Source: CAD feature listing. Evaluate the final solid. Frame: model axes, mm. A direction names the side the tool comes from. Give positions to 0.01 mm unless a question says otherwise; leave off trailing zeros. Order: outer loops, then holes, each group sorted by start corner. A loop starts at its lowest first (then second) coordinate and runs counter-clockwise, first axis right, second up. Notation, with made-up numbers: (76.5, 49.5) - (122.5, 49.5) arc R17 cw to (122.5, 82.5) - close; hole circle Ø4 at (28, -4). An arc over 180 degrees is marked (long way). Write each question's results on one line, items separated by ' | '. Start each with the question number.
Item 1: Section B-B on x = 1.1. Output: boundary loops of the cut face in (y, z).
Item 2: Set-up query: faces 5 (the flat face through (1, -52.5, 23)), 6 (the flat face through (1, -33, -20)). Return all of +Z, -Z, +X, -X, +Y, -Y with unobstructed straight access to the full face (end or side cutting, diameter ignored); none if empty.
Item 3: Section A-A on z = 0. Output: boundary loops of the cut face in (x, y).
Item 4: Section D-D on z = -6.5. Output: boundary loops of the cut face in (x, y), and give its area (3 significant figures).
Item 5: Contact query for flat-ended pins moving along their axis: pin 1 Ø3 at (y, z) = (0, 0) entering from -X; pin 2 Ø1.5 at (x, z) = (1.5, 10.5) entering from -Y. Output: stop coordinate, or through.
Item 6: Mould query, pull axis Z, two halves, no side actions, for faces 1 (the flat face through (1, -27, -25)), 2 (the flat face through (1, -26, 25)), 3 (the cylindrical face through (1.48, -2.44, 0.54)), 4 (the cylindrical face through (1.479, 24.994, -0.55)). Classes: released by +Z, released by -Z, zero draft, split by the parting line, or undercut.
Item 7: Section C-C on y = -33.5. Output: boundary loops of the cut face in (x, z).
Item 8: Line query: line 1 along Y through (x, z) = (2.25, 0); line 2 along Z through (x, y) = (2.2, -16); line 3 along Z through (x, y) = (0.65, -33). Output: solid intervals per line, ascending.
```python
from build123d import *

# Parameters (mm, degrees)
SKETCH1_R           = 2.5
BOSS_EXTRUDE1_DEPTH = 3


with BuildPart() as part:
    # Sketch1 → Boss-Extrude1 (new body)
    with BuildSketch(Plane(origin=(0, 0, 0), x_dir=(0, 0, -1), z_dir=(1, 0, 0))):
        with BuildLine():
            ThreePointArc((-20, -15), (-23.717082451, -7.90569415), (-25, 0))
            Line((-25, 0), (-25, -52.5))
            Line((-25, -52.5), (-20, -52.5))
            Line((-20, -52.5), (-20, -15))
        make_face()
        with BuildLine():
            ThreePointArc((25, 0), (0, 25), (-25, 0))
            ThreePointArc((-25, 0), (-23.717082451, -7.90569415), (-20, -15))
            ThreePointArc((-20, -15), (0, -25), (20, -15))
            ThreePointArc((20, -15), (23.717082451, -7.90569415), (25, 0))
        make_face()
        Circle(SKETCH1_R, mode=Mode.SUBTRACT)
        with BuildLine():
            Line((25, -52.5), (25, 0))
            ThreePointArc((25, 0), (23.717082451, -7.90569415), (20, -15))
            Line((20, -15), (20, -52.5))
            Line((20, -52.5), (25, -52.5))
        make_face()
    extrude(amount=BOSS_EXTRUDE1_DEPTH)


solid = part.part
```
Evaluation:
1) outline: (-52.5, -25) - (0, -25) arc R25 ccw to (0, 25) - (-52.5, 25) - (-52.5, 20) - (-15, 20) arc R25 ccw to (-15, -20) - (-52.5, -20) - close; hole circle Ø5 at (0, 0)
2) face 5: +Z, -Z, +X, -X, -Y | face 6: +X, -X, -Y
3) outline: (0, -25) - (3, -25) - (3, -2.5) - (0, -2.5) - close; (0, 2.5) - (3, 2.5) - (3, 25) - (0, 25) - close
4) outline: (0, -24.14) - (3, -24.14) - (3, 24.14) - (0, 24.14) - close | area: 145 mm^2
5) pin 1: passes through | pin 2: stops at y = -23.02
6) face 1: released by -Z | face 2: released by +Z | face 3: undercut | face 4: split by the parting line
7) outline: (0, -25) - (3, -25) - (3, -20) - (0, -20) - close; (0, 20) - (3, 20) - (3, 25) - (0, 25) - close
8) line 1: y = -25 to -2.5, 2.5 to 25 | line 2: z = -25 to -20, -19.21 to 19.21, 20 to 25 | line 3: z = -25 to -20, 20 to 25
